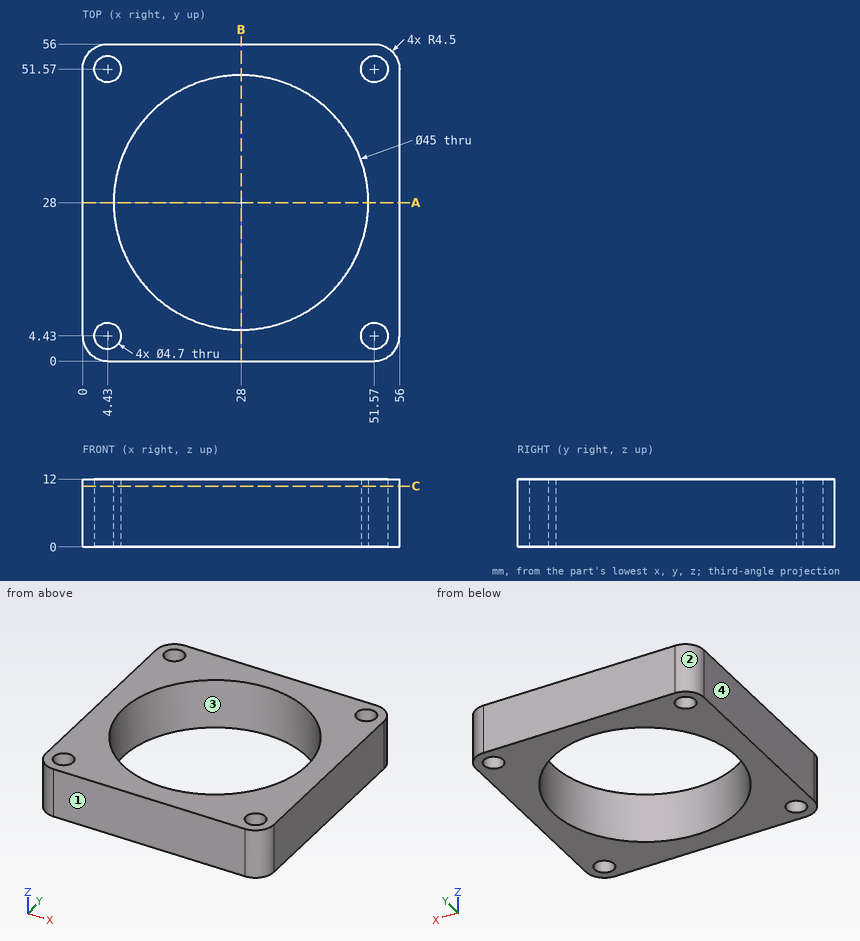
For this review, use the dimensioned drawing (mm, ordinates from the lowest corner) and the shaded views. Coordinates: 2 decimals unless noted, no trailing zeros. Order: outer loops, then holes, each group sorted by start corner. A loop starts at its lowest first (then second) coordinate and runs counter-clockwise, first axis right, second up. Notation, with made-up numbers: M 25.5,5.5 L 39.5,5.5 A20 ccw 39.5,27.5 Z; hole C 62,-21.75 d11. An arc over 180 degrees is marked long. Answer as a JSON object with one key per item and string values. Group by question number.
1) Mouldability with a two-part tool opening along Y and no side actions: class the marked faces 1, 2, 3 and 4 as pulls with the +Y half, pulls with the -Y half, needs draft (parallel to the pull), parting line crosses it, or undercut.
2) Wall thickness on L1, parallel to Y at x = 4.43, z = 6.75; L2, parallel to Y at x = 28, z = 9; L3, parallel to Y at x = 52, z = 10.5: over which ranges is each line inside the solid? List them lowest first.
3) Add section A-A, the plane y = 28. Write out the cut boundary in (x, z).
4) Add section C-C, the plane z = 10.75. Write out the cut boundary in (x, y), then the cut area to 3 significant figures.
Computed values:
{
 "1": {"face 1": "pulls with the -Y half", "face 2": "pulls with the +Y half", "face 3": "undercut", "face 4": "needs draft"},
 "2": {"L1": "y = 0 to 2.08, 6.78 to 49.22, 53.92 to 56", "L2": "y = 0 to 5.5, 50.5 to 56", "L3": "y = 0.03 to 2.12, 6.74 to 49.26, 53.88 to 55.97"},
 "3": {"outline": "M 0,0 L 5.5,0 L 5.5,12 L 0,12 Z; M 50.5,0 L 56,0 L 56,12 L 50.5,12 Z"},
 "4": {"outline": "M 0,4.5 A4.5 ccw 4.5,0 L 51.5,0 A4.5 ccw 56,4.5 L 56,51.5 A4.5 ccw 51.5,56 L 4.5,56 A4.5 ccw 0,51.5 Z; hole C 4.43,4.43 d4.7; hole C 4.43,51.57 d4.7; hole C 28,28 d45; hole C 51.57,4.43 d4.7; hole C 51.57,51.57 d4.7", "area": "1,460 mm^2"}
}
